Can you work these out from the model? Positions are in its coordinate system, mm. A direction names the side the tool comes from. Round coordinates to 2 decimals unless told otherwise and drop trailing zeros. Order: outer loops, then holes, each group sorted by start corner. A loop starts at its lowest first (then second) coordinate and runs counter-clockwise, first axis right, second up. Notation, with made-up numbers: (45.5, 44) -> (95.5, 44) arc R17 cw to (95.5, 50) -> close; hole circle Ø7 at (-6.75, 20). An arc over 180 degrees is marked (long way). One line per item, written item: value.
```python
from build123d import *

# Parameters (mm, degrees)
EXTRUDE_1_DEPTH = 50
SKETCH_3_R      = 2.5
EXTRUDE_2_DEPTH = 10
FILLET_1_R      = 20


with BuildPart() as part:
    # Эскиз2 → Бобышка-Вытянуть1 (new body)
    with BuildSketch(Plane(origin=(0, 0, 0), x_dir=(1, 0, 0), z_dir=(0, 1, 0))):
        with BuildLine():
            Line((20.775320905, -61.764467554), (20.775320905, -69.224273938))
            ThreePointArc((20.775320905, -69.224273938), (16.381922622, -79.830875656), (5.775320905, -84.224273938))
            Line((5.775320905, -84.224273938), (1.80486375, -84.224273938))
            ThreePointArc((1.80486375, -84.224273938), (-8.801737968, -79.830875656), (-13.19513625, -69.224273938))
            Line((-13.19513625, -69.224273938), (-13.19513625, 60.360729655))
            Line((-13.19513625, 60.360729655), (20.775320905, 60.360729655))
            Line((20.775320905, 60.360729655), (20.775320905, 17.687097527))
            ThreePointArc((20.775320905, 17.687097527), (7.863671927, -22.038685014), (20.775320905, -61.764467554))
        make_face()
    extrude(amount=EXTRUDE_1_DEPTH)

    # Эскиз3 → Бобышка-Вытянуть2 (add)
    with BuildSketch(Plane(origin=(0, 50, 0), x_dir=(1, 0, 0), z_dir=(0, 1, 0))):
        with Locations(Location((3.403106264, 42.800743613, 0), (0, 0, 270))):
            Circle(SKETCH_3_R)
    extrude(amount=EXTRUDE_2_DEPTH)

    # Скругление1
    # the kernel refuses this fillet: 20 mm, written as the material it takes off along each edge
    with BuildSketch(Plane(origin=(-13.19513625, -50, -60.360729655), x_dir=(0, 0, 1), z_dir=(0, 1, 0))) as fillet_1_piece_1:
        with BuildLine():
            CenterArc((FILLET_1_R, FILLET_1_R), FILLET_1_R, 180, 90)
            Line((0, FILLET_1_R), (0, 0))
            Line((0, 0), (FILLET_1_R, 0))
        make_face()
    extrude(amount=150, mode=Mode.SUBTRACT)
    with BuildSketch(Plane(origin=(20.775320905, -50, -60.360729655), x_dir=(0, 0, 1), z_dir=(0, 1, 0))) as fillet_1_piece_2:
        with BuildLine():
            CenterArc((FILLET_1_R, -FILLET_1_R), FILLET_1_R, 90, 90)
            Line((0, -FILLET_1_R), (0, 0))
            Line((0, 0), (FILLET_1_R, 0))
        make_face()
    extrude(amount=150, mode=Mode.SUBTRACT)


solid = part.part
```
Q1. Will these pins go through, and if not, where does the flat tip stop? pin 1 Ø1 at (x, y) = (15.5, 8.5) entering from -Z; pin 2 Ø3 at (x, y) = (-6.5, 28) entering from -Z; pin 3 Ø4 at (x, z) = (0, 65) entering from +Y.
Answers below:
pin 1: z = -54.42
pin 2: z = -56.51
pin 3: y = 50
Q2. On a 3-axis mill with a long thin cutter (end or side, diameter ignored), from which of +Z, -Z, +X, -X, +Y, -Y can I reach the whole of each face in a straight line? I mean faces 1 (the face through (20.775, 25, -29)), 2 (the face through (3.5, 54.9, -45.3)). Say none if no direction works.
Answers below:
face 1: +Z, -Z, +X, +Y, -Y
face 2: +Y
Q3. I want a section at D-D on x = 11.5. List the corners of the cut face in (y, z) for me.
Answers below:
outline: (0, -57.24) -> (50, -57.24) -> (50, 0.17) -> (0, 0.17) -> close; (0, 43.91) -> (50, 43.91) -> (50, 83.09) -> (0, 83.09) -> close
Q4. I want a section at C-C on z = 66. List the corners of the cut face in (x, y) for me.
Answers below:
outline: (-13.2, 0) -> (20.78, 0) -> (20.78, 50) -> (-13.2, 50) -> close
Q5. Please list where these lines run through material, in increasing order: line 1 along Y through (x, z) = (9, -35); line 2 along Z through (x, y) = (19, 5); line 3 along X through (y, z) = (38.5, 69.5).
Answers below:
line 1: 0 to 50
line 2: -48.6 to -15.12, 59.2 to 76.3
line 3: -13.19 to 20.77
Q6. I want a section at B-B on y = 35. List the corners of the cut face in (x, z) for me.
Answers below:
outline: (-13.2, -40.36) arc R20 ccw to (3.79, -60.13) arc R20 ccw to (20.78, -40.36) -> (20.78, -17.69) arc R67.57 cw to (20.78, 61.76) -> (20.78, 69.22) arc R15 ccw to (5.78, 84.22) -> (1.8, 84.22) arc R15 ccw to (-13.2, 69.22) -> close
Q7. I want a section at A-A on x = 17.5. List the corners of the cut face in (y, z) for me, plus the area to 3 significant figures.
Answers below:
outline: (0, -51.33) -> (50, -51.33) -> (50, -12.74) -> (0, -12.74) -> close; (0, 56.81) -> (50, 56.81) -> (50, 78.58) -> (0, 78.58) -> close
area: 3,020 mm^2
